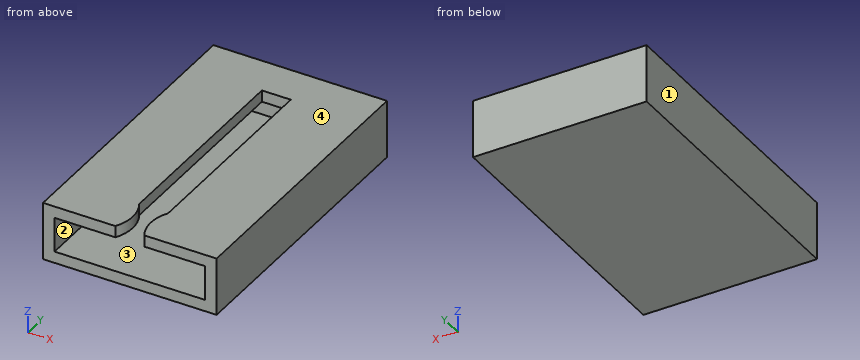
from build123d import *

# Parameters (mm, degrees)
F0_W     = 38.1
F0_H     = 63.5
F1_DEPTH = 12.7
F2_T     = -2.54
F3_W     = 6.35
F3_H     = 45.72
F4_DEPTH = 2.54


with BuildPart() as f1:
    # F0 (on Top) → F1 (new body)
    with BuildSketch(Plane.XY):
        Rectangle(F0_W, F0_H)
    extrude(amount=F1_DEPTH)

    # F2
    f2_openings = [f1.faces().sort_by_distance(p)[0] for p in [
        (0, -31.75, 6.35),
    ]]
    offset(amount=F2_T, openings=f2_openings)

    # F3 (on face) → F4 (cut, through all)
    with BuildSketch(Plane.XY.offset(12.7)):
        Rectangle(F3_W, F3_H)
        with BuildLine():
            ThreePointArc((3.175, -31.75), (1.976942, -27.305), (3.175, -22.86))
            Line((3.175, -22.86), (-3.175, -22.86))
            ThreePointArc((-3.175, -22.86), (-1.976942, -27.305), (-3.175, -31.75))
            Line((-3.175, -31.75), (3.175, -31.75))
        make_face()
    extrude(amount=-F4_DEPTH, mode=Mode.SUBTRACT)


solid = f1.part
Source: CAD feature listing. Evaluate the final solid. Frame: model axes, mm. Face numbers are marked on the shaded views. Round coordinates to 2 decimals unless told otherwise and drop trailing zeros. Loops run counter-clockwise (first coordinate to the right, second up) from the corner with the lowest first, then second, coordinate; pieces in that order, holes last. Notation, with made-up numbers: M 79,54.25 L 121,54.25 A12 cw 121,71.25 Z; hole C 42.25,27.25 d5. An arc over 180 degrees is marked long. Return JSON: item names as keys, results as strings. Group by question number.
1. Section query C-C on y = -13. Output: boundary loops of the cut face in (x, z) (3 decimals), and give its area (3 significant figures).
2. Mould query, pull axis X, two halves, no side actions, for the marked faces 1, 2, 3 and 4. Classes: released by +X, released by -X, zero draft, split by the parting line, or undercut.
3. Section query A-A on y = 27.5. Output: boundary loops of the cut face in (x, z).
4. Pin query (flat end, axial travel): pin 1 (1.3 mm diameter, centred on x = 0, z = 12, fed in from -Y); pin 2 (5 mm diameter, centred on x = 1, z = 7.5, fed in from -Y). Return the tip coordinate at first contact, or that it passes through.
5. Material intervals for line 1 along X through (y, z) = (-16, 6.25); line 2 along Z through (x, y) = (-9.5, 23.5); line 3 along X through (y, z) = (-13, 11.75) (3 decimals), sorted ascending. Write a range as from..to.
6. Section query D-D on z = 5.25. Output: boundary loops of the cut face in (x, y), and give its area (3 significant figures).
7. Section query B-B on x = 9. Output: boundary loops of the cut face in (y, z), and give its area (3 significant figures).
Checks:
{
 "1": {"outline": "M -19.05,0 L 19.05,0 L 19.05,12.7 L 3.175,12.7 L 3.175,10.16 L 16.51,10.16 L 16.51,2.54 L -16.51,2.54 L -16.51,10.16 L -3.175,10.16 L -3.175,12.7 L -19.05,12.7 Z", "area": "216 mm²"},
 "2": {"face 1": "released by -X", "face 2": "undercut", "face 3": "undercut", "face 4": "zero draft"},
 "3": {"outline": "M -19.05,0 L 19.05,0 L 19.05,12.7 L -19.05,12.7 Z; hole M -16.51,2.54 L 16.51,2.54 L 16.51,10.16 L -16.51,10.16 Z"},
 "4": {"pin 1": "stops at y = 22.86", "pin 2": "stops at y = 29.21"},
 "5": {"line 1": "x = -19.05..-16.51, 16.51..19.05", "line 2": "z = 0..2.54, 10.16..12.7", "line 3": "x = -19.05..-3.175, 3.175..19.05"},
 "6": {"outline": "M -19.05,-31.75 L -16.51,-31.75 L -16.51,29.21 L 16.51,29.21 L 16.51,-31.75 L 19.05,-31.75 L 19.05,31.75 L -19.05,31.75 Z", "area": "406 mm²"},
 "7": {"outline": "M -31.75,0 L 31.75,0 L 31.75,12.7 L -31.75,12.7 L -31.75,10.16 L 29.21,10.16 L 29.21,2.54 L -31.75,2.54 Z", "area": "342 mm²"}
}
